from build123d import *

# Parameters (mm, degrees)
F0_R     = 38.1
F0_R_2   = 25.4
F1_DEPTH = 3.175
F2_R     = 1.27
F3_R     = 1.27


# Not quite as in the source:
# - a fillet or chamfer that OpenCascade refuses, or shapes differently, is made with other operations: its cross-section is extruded or revolved along the edge and cut away or added


with BuildPart() as f1:
    # F0 (on Front) → F1 (new body)
    with BuildSketch(Plane.XZ):
        Circle(F0_R)
        Circle(F0_R_2, mode=Mode.SUBTRACT)
    extrude(amount=F1_DEPTH)

    # F2
    f2_edges = [f1.edges().sort_by_distance(p)[0] for p in [
        (-25.4, 0, 0),
        (-25.4, -3.175, 0),
    ]]
    fillet(f2_edges, radius=F2_R)

    # F4: chamfer of 3.81 on 1 edges, made by hand

    # F4_s1 → F4_t2 (revolve, cut)
    with BuildSketch(Plane.XY):
        Polygon((34.29, -3.175), (38.1, 0.635), (38.1, -3.175), align=None)
    revolve(axis=Axis((0, -3.175, 0), (0, -1, 0)), mode=Mode.SUBTRACT)

    # F3
    f3_edges = [f1.edges().sort_by_distance(p)[0] for p in [
        (-34.29, -3.175, 0),
    ]]
    fillet(f3_edges, radius=F3_R)


solid = f1.part
Geometry: final body of the model. Coordinates: model frame, mm. Give positions to 0.01 mm unless a question says otherwise; leave off trailing zeros. Loops run counter-clockwise (first coordinate to the right, second up) from the corner with the lowest first, then second, coordinate; pieces in that order, holes last. Notation, with made-up numbers: (31.25, 16.25) - (69.25, 16.25) arc R32 cw to (69.25, 52.25) - close; hole circle Ø2 at (3, -17). An arc over 180 degrees is marked (long way). One line per question, with ' | ' between items. Start each with the question number.
(1) Pull-direction query (Z, two-part tool) for faces 1 (the cylindrical face through (-5.506, -1.583, -24.796)), 2 (the conical face through (33.23, -2.63, 10.46)), 3 (the flat face through (25, -3.175, 10)); classes: released by +Z, released by -Z, zero draft, split by the parting line, or undercut.
(2) Contact query for a flat-ended pin moving along its axis: pin 1 (1 mm diameter, centred on y = -2, z = 13, fed in from -X). Output: stop coordinate, or through.
(3) Section query C-C on y = -0.5. Return loops of the section in (x, z) (3 decimals).
(4) Section query A-A on z = 0. Return loops of the section in (x, y) (3 decimals), then the cut area to 3 significant figures.
(5) Section query B-B on x = 0. Return loops of the section in (y, z) (3 decimals).
(6) Ray query, line 1 (X direction, y = -1.55, z = -4); line 2 (Z direction, x = 0, y = -1.45) (3 decimals); line 3 (Z direction, x = 18.5, y = -2.4). Return the intervals inside material, ascending. Write a range as from..to.
The answers:
1) face 1: undercut | face 2: split by the parting line | face 3: zero draft
2) pin 1: x = -33.57
3) outline: circle Ø73.93 at (0, 0); hole circle Ø51.32 at (0, 0)
4) outline: (-37.465, 0) - (-34.662, -2.803) arc R1.27 ccw to (-33.764, -3.175) - (-26.67, -3.175) arc R1.27 ccw to (-25.4, -1.905) - (-25.4, -1.27) arc R1.27 ccw to (-26.67, 0) - close; (25.4, -1.905) arc R1.27 ccw to (26.67, -3.175) - (33.764, -3.175) arc R1.27 ccw to (34.662, -2.803) - (37.465, 0) - (26.67, 0) arc R1.27 ccw to (25.4, -1.27) - close | area: 65.1 mm2
5) outline: (-3.175, -33.764) arc R1.27 ccw to (-2.803, -34.662) - (0, -37.465) - (0, -26.67) arc R1.27 ccw to (-1.27, -25.4) - (-1.905, -25.4) arc R1.27 ccw to (-3.175, -26.67) - close; (-3.175, 26.67) arc R1.27 ccw to (-1.905, 25.4) - (-1.27, 25.4) arc R1.27 ccw to (0, 26.67) - (0, 37.465) - (-2.803, 34.662) arc R1.27 ccw to (-3.175, 33.764) - close
6) line 1: -35.69..-25.08, 25.08..35.69 | line 2: -36.015..-25.4, 25.4..36.015 | line 3: -29.79..-17.55, 17.55..29.79
